```python
from build123d import *

# Parameters (mm, degrees)
BOSS_EXTRUDE1_DEPTH     = 2.5
SKETCH4_R               = 0.35
THROUGH_HOLES_DEPTH     = 4.688156721
FILLET1_R               = 0.125
SKETCH5_R               = 0.125
BOSS_EXTRUDE2_DEPTH     = 0.5
SKETCH8_R               = 0.46
CUT_EXTRUDE1_DEPTH      = 5.582575695
CUT_EXTRUDE2_DEPTH      = 5.562071898
CUT_EXTRUDE2_DEPTH_BACK = 5.562071898
SKETCH9_W               = 1.465031661
SKETCH9_H               = 4
BOSS_EXTRUDE3_DEPTH     = 1.75


with BuildPart() as part:
    # Sketch3 → Boss-Extrude1 (new body)
    with BuildSketch(Plane(origin=(0, 0, 0), x_dir=(1, 0, 0), z_dir=(0, 1, 0))):
        with BuildLine():
            Line((-2.5, 0.9), (-2, 0.93))
            Line((-2, 0.93), (-2, 0.56))
            Line((-2, 0.56), (-1.5, 0.56))
            Line((-1.5, 0.56), (-1.5, 0.96))
            Line((-1.5, 0.96), (0, 1.05))
            ThreePointArc((0, 1.05), (1.05, 0), (0, -1.05))
            Line((0, -1.05), (-1.5, -0.96))
            Line((-1.5, -0.96), (-1.5, -0.56))
            Line((-1.5, -0.56), (-2, -0.56))
            Line((-2, -0.56), (-2, -0.93))
            Line((-2, -0.93), (-2.5, -0.9))
            Line((-2.5, -0.9), (-2.5, 0.9))
        make_face()
    extrude(amount=BOSS_EXTRUDE1_DEPTH)

    # Sketch4 → Through Holes (cut, through all)
    with BuildSketch(Plane(origin=(0, 2.5, 0), x_dir=(1, 0, 0), z_dir=(0, 1, 0))):
        with Locations(Location((0, 0, 0), (0, 0, 270))):
            Circle(SKETCH4_R)
    extrude(amount=-THROUGH_HOLES_DEPTH, mode=Mode.SUBTRACT)

    # Fillet1
    fillet1_edges = [part.edges().sort_by_distance(p)[0] for p in [
        (-2, 1.25, -0.56),
        (-1.5, 1.25, -0.56),
        (-1.5, 1.25, 0.56),
        (-2, 1.25, 0.56),
    ]]
    fillet(fillet1_edges, radius=FILLET1_R)

    # Sketch5 → Boss-Extrude2 (add)
    with BuildSketch(Plane(origin=(0, 0, 0), x_dir=(1, 0, 0), z_dir=(0, 1, 0))):
        Polygon((-2.25, -2), (1.75, -2), (3.25, -2), (3.25, 2), (1.75, 2), (-2.25, 2), align=None)
        with Locations(Location((0, 0, 0), (0, 0, 270))):
            Circle(SKETCH5_R, mode=Mode.SUBTRACT)
    extrude(amount=-BOSS_EXTRUDE2_DEPTH)

    # Sketch8 → Cut-Extrude1 (cut, through all)
    with BuildSketch(Plane(origin=(0.7, 2.1, 0), x_dir=(0.948683298050514, -0.3162277660168378, 0), z_dir=(0.3162277660168378, 0.948683298050514, 0))):
        with Locations((1.987936011, 0)):
            Circle(SKETCH8_R)
    extrude(amount=-CUT_EXTRUDE1_DEPTH, mode=Mode.SUBTRACT)

    # Sketch9 → Cut-Extrude2 (cut, two sides: drawn at the far end of the back side and taken through both)
    with BuildSketch(Plane.XZ.offset(-CUT_EXTRUDE2_DEPTH_BACK)):
        with Locations((-2.982515831, 0)):
            Rectangle(SKETCH9_W, SKETCH9_H)
    extrude(amount=CUT_EXTRUDE2_DEPTH + CUT_EXTRUDE2_DEPTH_BACK, mode=Mode.SUBTRACT)

    # Sketch10 → Boss-Extrude3 (add)
    with BuildSketch(Plane.XZ.offset(0.5)):
        Polygon((-1.5, 1.25), (-1.5, -1.25), (-0.75, -1.25), (0, 0), (-0.75, 1.25), align=None)
    extrude(amount=BOSS_EXTRUDE3_DEPTH)


solid = part.part
```
Read the model definition and answer for the solid it produces. Units are mm, in the model's axes. A direction names the side the tool comes from. Round coordinates to 2 decimals unless told otherwise and drop trailing zeros. Write each loop counter-clockwise with the first axis right and the second up, starting at its lowest first coordinate (ties: lowest second). Pieces come first, ordered by that corner, then holes. Notation, with made-up numbers: (76, 5) - (101, 5) arc R25 cw to (101, 42) - close; hole circle Ø6 at (83, 23.25). An arc over 180 degrees is marked (long way). Use CSV: the item, a comma, the result in double quotes.
Q1. Find section C-C, the plane x = -0.85. Write down the section's boundary in (y, z).
Values:
outline,"(-2.25, -1.25) - (-0.5, -1.25) - (-0.5, -2) - (0, -2) - (0, -1) - (2.5, -1) - (2.5, 1) - (0, 1) - (0, 2) - (-0.5, 2) - (-0.5, 1.25) - (-2.25, 1.25) - close"
Q2. Find section B-B, the plane y = -1.2. Write down the section's boundary in (x, z).
Values:
outline,"(-1.5, -1.25) - (-0.75, -1.25) - (0, 0) - (-0.75, 1.25) - (-1.5, 1.25) - close"
Q3. Find section D-D, the plane y = -0.15. Count the separate pieces of the cut face and the enclosed holes in it, then the cut area to 3 significant figures.
Values:
separate pieces,"1"
enclosed holes,"2"
area,"21.3 mm²"
Q4. Straight lines are drawn through the part: line 1 along Z through (x, y) = (0, -0.2) (3 decimals); line 2 along X through (y, z) = (1, 0); line 3 along X through (y, z) = (-0.3, 0) (3 decimals). For each, find the intervals that lie inside material, in ascending order.
Values:
line 1,"z = -2 to -0.125, 0.125 to 2"
line 2,"x = -2.25 to -0.35, 0.35 to 1.05"
line 3,"x = -2.25 to -0.125, 0.125 to 1.511, 2.48 to 3.25"
Q5. Find section A-A, the plane y = 2.1. Write down the section's boundary in (x, z) (3 decimals).
Values:
outline,"(-2.25, -0.915) - (-2, -0.93) - (-2, -0.685) arc R0.125 cw to (-1.875, -0.56) - (-1.625, -0.56) arc R0.125 cw to (-1.5, -0.685) - (-1.5, -0.96) - (0, -1.05) arc R1.05 ccw to (0, 1.05) - (-1.5, 0.96) - (-1.5, 0.685) arc R0.125 cw to (-1.625, 0.56) - (-1.875, 0.56) arc R0.125 cw to (-2, 0.685) - (-2, 0.93) - (-2.25, 0.915) - close; hole circle Ø0.7 at (0, 0)"
Q6. Determine the mould class of faces 1 (the flat face through (-1, -2.25, 0)), 2 (the flat face through (-0.74, 1.232, 1.006)), 3 (the cylindrical face through (2.21, -0.32, 0.41)) for opening direction X: +X half, -X half, draft (parallel to the pull), parting line (faces both ways), or undercut.
Values:
face 1,"draft"
face 2,"-X half"
face 3,"undercut"
Q7. Each of these flat-tipped pins is pushed along its axis until it touches: pin 1 Ø0.6 at (x, y) = (-1, -1.5) entering from -Z; pin 2 Ø0.9 at (y, z) = (-1.5, 0) entering from -X. Where does it stop, or does it pass through?
Values:
pin 1,"stops at z = -1.25"
pin 2,"stops at x = -1.5"
Q8. A tool of negligible diameter and unlimited length cuts with its end or side. For faces 4 (the flat face through (-1.5, -1, 0)), 5 (the flat face through (-0.38, -1.36, -0.63)), 6 (the flat face through (-0.8, 1.2, -1)), 7 (the flat face through (-0.37, -1.36, 0.62)), 8 (the cylindrical face through (1.05, 1.23, -0.02)), from which of +Z, -Z, +X, -X, +Y, -Y can it reach the whole face along a straight path? Write none if from no direction.
Values:
face 4,"+Z, -Z, -X, -Y"
face 5,"-Z, +X, -Y"
face 6,"-Z, -X, +Y"
face 7,"+Z, +X, -Y"
face 8,"+X, +Y"
